For this review, take the finished solid that the model builds, in its own axes (mm). Face numbers are marked on the shaded views. A direction names the side the tool comes from. Give positions to 0.01 mm unless a question says otherwise; leave off trailing zeros. Order: outer loops, then holes, each group sorted by start corner. A loop starts at its lowest first (then second) coordinate and runs counter-clockwise, first axis right, second up. Notation, with made-up numbers: (-18.75, 52) -> (12.25, 52) arc R22 ccw to (12.25, 75) -> close; hole circle Ø1 at (-27.5, -37). An arc over 180 degrees is marked (long way). One line per item, written item: value. Start each with the question number.
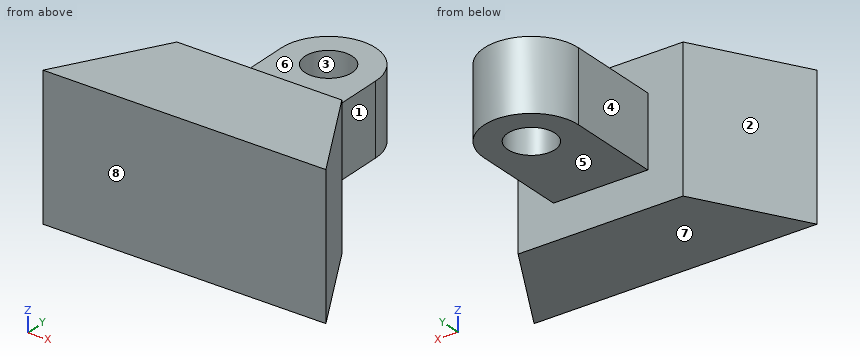
from build123d import *

# Parameters (mm, degrees)
Y_KSEKLIK_EKSTR_ZYON1_DEPTH = 30
IZIM2_R                     = 10
Y_KSEKLIK_EKSTR_ZYON2_DEPTH = 15


with BuildPart() as part:
    # Çizim1 → Yükseklik-Ekstrüzyon1 (new, symmetric)
    with BuildSketch(Plane.XY):
        Polygon((-60, -21.650635095), (60, -21.650635095), (35, 21.650635095), (-35, 21.650635095), align=None)
    extrude(amount=Y_KSEKLIK_EKSTR_ZYON1_DEPTH, both=True)

    # Çizim2 → Yükseklik-Ekstrüzyon2 (add, symmetric)
    with BuildSketch(Plane.XY):
        with BuildLine():
            Line((-20, 21.650635095), (-20, 61.650635095))
            ThreePointArc((-20, 61.650635095), (0, 81.650635095), (20, 61.650635095))
            Line((20, 61.650635095), (20, 21.650635095))
            Line((20, 21.650635095), (-20, 21.650635095))
        make_face()
        with Locations((0, 61.650635095)):
            Circle(IZIM2_R, mode=Mode.SUBTRACT)
    extrude(amount=Y_KSEKLIK_EKSTR_ZYON2_DEPTH, both=True)


solid = part.part
Q1. Take a section at B-B (x = 0). State the section outline as (y, z) points, and give its area (3 significant figures).
Q2. Take a section at D-D (z = 20). State the section outline as (x, y) points.
Q3. For the marked faces 4, 5, 6, 7 and 8, list the 3-axis set-ups (+Z, -Z, +X, -X, +Y, -Y) from which the entire face can be reached by the end or side of a thin tool; tool diameter is ignored.
Q4. For pin 1 Ø24 at (y, z) = (37.5, -7) entering from +X; pin 2 Ø8 at (x, y) = (-19, 61) entering from +Z; pin 3 Ø5 at (x, z) = (-17, 10.5) entering from +Y, all flat-tipped, find the tip position at first contact; note any pin that passes through.
Q5. Mouldability with a two-part tool opening along Y and no side actions: class the marked faces 1, 2 and 3 as pulls with the +Y half, pulls with the -Y half, needs draft (parallel to the pull), parting line crosses it, or undercut.
Q6. Take a section at A-A (z = -2.5). State the section outline as (x, y) points.
Q7. For line 1 along Y through (x, z) = (0, -3.5); line 2 along X through (y, z) = (46, 12.5); line 3 along Y through (x, z) = (3, 18.5), list the stretches that pass through material, from the lowest coordinate up.
Q8. Take a section at C-C (y = 65). State the section outline as (x, z) points.
Answers below:
1. outline: (-21.65, -30) -> (21.65, -30) -> (21.65, -15) -> (51.65, -15) -> (51.65, 15) -> (21.65, 15) -> (21.65, 30) -> (-21.65, 30) -> close; (71.65, -15) -> (81.65, -15) -> (81.65, 15) -> (71.65, 15) -> close
1. area: 3,800 mm²
2. outline: (-60, -21.65) -> (60, -21.65) -> (35, 21.65) -> (-35, 21.65) -> close
3. face 4: +Z, -Z, -X, +Y
3. face 5: -Z, +X, -X, +Y
3. face 6: +Z, +X, -X, +Y
3. face 7: -Z, +X, -X, +Y, -Y
3. face 8: +Z, -Z, +X, -X, -Y
4. pin 1: stops at x = 20
4. pin 2: stops at z = 15
4. pin 3: stops at y = 75.43
5. face 1: needs draft
5. face 2: pulls with the +Y half
5. face 3: undercut
6. outline: (-60, -21.65) -> (60, -21.65) -> (35, 21.65) -> (20, 21.65) -> (20, 61.65) arc R20 ccw to (-20, 61.65) -> (-20, 21.65) -> (-35, 21.65) -> close; hole circle Ø20 at (0, 61.65)
7. line 1: y = -21.65 to 51.65, 71.65 to 81.65
7. line 2: x = -20 to 20
7. line 3: y = -21.65 to 21.65
8. outline: (-19.72, -15) -> (-9.42, -15) -> (-9.42, 15) -> (-19.72, 15) -> close; (9.42, -15) -> (19.72, -15) -> (19.72, 15) -> (9.42, 15) -> close
